Answer from the drawing. Dimensions are ordinates in mm from the lowest x, y and z of the part. Give positions to 0.01 mm unless a question says otherwise; leave off trailing zeros. Loops run counter-clockwise (first coordinate to the right, second up) from the corner with the lowest first, then second, coordinate; pieces in that order, holes last.
Item 1: Section B-B, the plane z = 430 is taken. Give the vertices of the cut face in (x, y).
Item 2: Consider line 1 along X through (y, z) = (7.5, 150); line 2 along Z through (x, y) = (102, 11.5); line 3 along X through (y, z) = (20.25, 430). Determine where each line is inside the solid, lowest interval first.
Item 3: Section A-A, the plane x = 100 is taken. Give the vertices of the cut face in (y, z), and give its area (3 significant figures).
Item 4: Each of these flat-tipped pins is pushed along its axis until it touches: pin 1 Ø25 at (x, z) = (782, 427.5) entering from -Y; pin 2 Ø25 at (x, z) = (107.5, 144) entering from -Y. Where does it stop, or does it pass through?
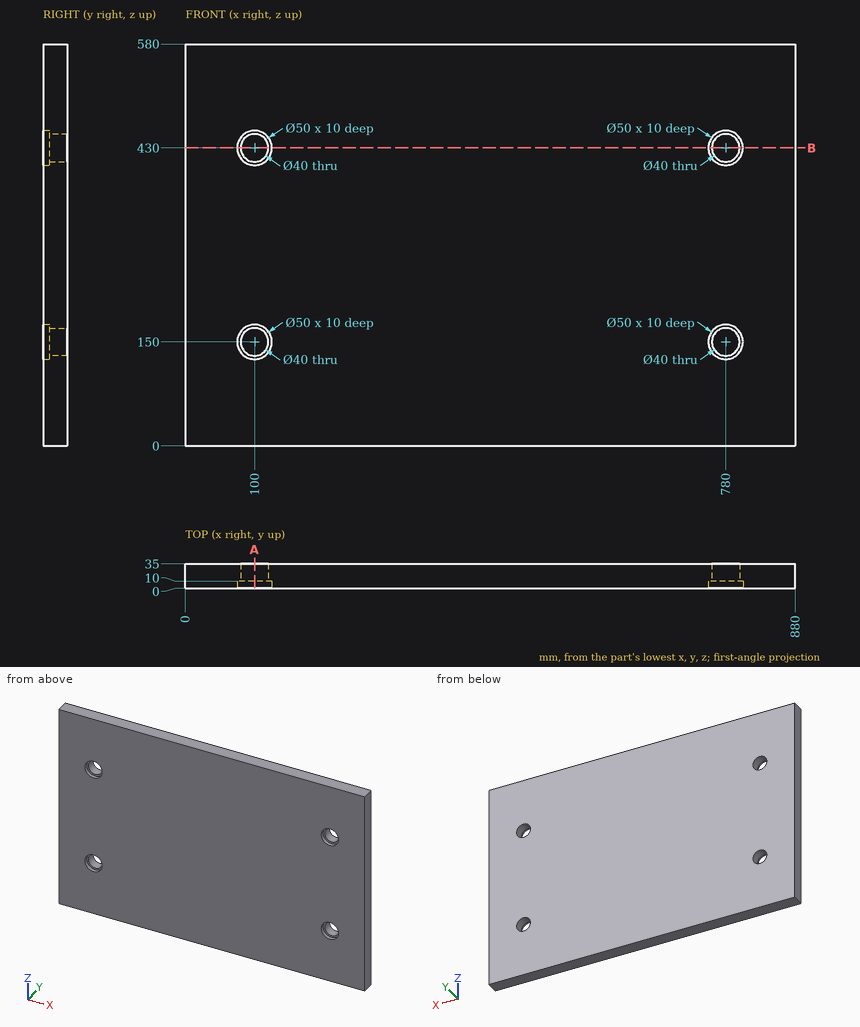
Worked answers:
1. outline: (0, 0) - (75, 0) - (75, 10) - (80, 10) - (80, 35) - (0, 35) - close; (120, 10) - (125, 10) - (125, 0) - (755, 0) - (755, 10) - (760, 10) - (760, 35) - (120, 35) - close; (800, 10) - (805, 10) - (805, 0) - (880, 0) - (880, 35) - (800, 35) - close
2. line 1: x = 0 to 75, 125 to 755, 805 to 880
2. line 2: z = 0 to 130.1, 169.9 to 410.1, 449.9 to 580
2. line 3: x = 0 to 80, 120 to 760, 800 to 880
3. outline: (0, 0) - (35, 0) - (35, 130) - (10, 130) - (10, 125) - (0, 125) - close; (0, 175) - (10, 175) - (10, 170) - (35, 170) - (35, 410) - (10, 410) - (10, 405) - (0, 405) - close; (0, 455) - (10, 455) - (10, 450) - (35, 450) - (35, 580) - (0, 580) - close
3. area: 17,300 mm2
4. pin 1: passes through
4. pin 2: stops at y = 10
